Read the model definition and answer for the solid it produces. Units are mm, in the model's axes. Coordinates: 2 decimals unless noted, no trailing zeros. Loops run counter-clockwise (first coordinate to the right, second up) from the corner with the lowest first, then second, coordinate; pieces in that order, holes last.
from build123d import *

# Parameters (mm, degrees)
F0_R     = 5
F1_DEPTH = 10
F2_R     = 2.5
F3_DEPTH = 25
F4_R     = 2.5
F5_DEPTH = 25
F0_R_2   = 2.5
F6_DEPTH = 3


with BuildPart() as f1:
    # F0 (on Front) → F1 (new body)
    with BuildSketch(Plane.XZ):
        with BuildLine():
            Line((-75, 45), (-85, 45))
            Line((-85, 45), (-85, -45))
            Line((-85, -45), (-75, -45))
            Line((-75, -45), (-75, -35))
            Line((-75, -35), (85.1359899874, -35.6216732085))
            ThreePointArc((85.1359899874, -35.6216732085), (120, -0.6219373992), (85.1359899874, 34.3777984101))
            Line((85.1359899874, 34.3777984101), (-75, 35))
            Line((-75, 35), (-75, 45))
        make_face()
        with BuildLine():
            ThreePointArc((87.5, -12.6219373992), (83.232233047, -14.3897043522), (85, -10.1219373992))
            ThreePointArc((85, -10.1219373992), (86.767766953, -10.8541704462), (87.5, -12.6219373992))
        make_face(mode=Mode.SUBTRACT)
        with BuildLine():
            ThreePointArc((85, 3.3780626008), (87.8284271247, 2.2064897255), (89, -0.6219373992))
            ThreePointArc((89, -0.6219373992), (87.8284271247, -3.450364524), (85, -4.6219373992))
            ThreePointArc((85, -4.6219373992), (81, -0.6219373992), (85, 3.3780626008))
        make_face(mode=Mode.SUBTRACT)
        with Locations((-75, 0)):
            Circle(F0_R, mode=Mode.SUBTRACT)
        Circle(F0_R, mode=Mode.SUBTRACT)
        with BuildLine():
            ThreePointArc((87.5, 11.3780626008), (86.767766953, 9.6102956478), (85, 8.8780626008))
            ThreePointArc((85, 8.8780626008), (83.232233047, 13.1458295538), (87.5, 11.3780626008))
        make_face(mode=Mode.SUBTRACT)
    extrude(amount=F1_DEPTH)

    # F2 (on face) → F3 (cut)
    with BuildSketch(Plane.YZ.offset(-75)):
        with Locations((-5, 40)):
            Circle(F2_R)
    extrude(amount=-F3_DEPTH, mode=Mode.SUBTRACT)

    # F4 (on face) → F5 (cut)
    with BuildSketch(Plane.YZ.offset(-75)):
        with Locations((-5, -40)):
            Circle(F4_R)
    extrude(amount=-F5_DEPTH, mode=Mode.SUBTRACT)

    # F0 (on Front) → F6 (join)
    with BuildSketch(Plane.XZ):
        with Locations((-75, 0)):
            Circle(F0_R)
        with Locations((-75, 0)):
            Circle(F0_R_2, mode=Mode.SUBTRACT)
        Circle(F0_R)
        Circle(F0_R_2, mode=Mode.SUBTRACT)
    extrude(amount=F6_DEPTH)


solid = f1.part
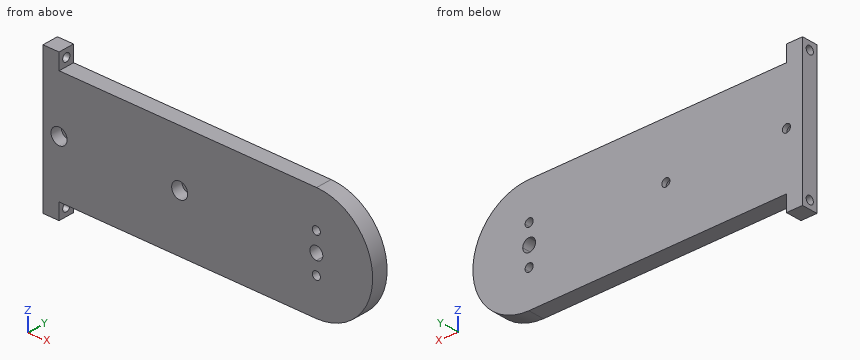
Item 1: Given pin 1 (12 mm diameter, centred on x = 25.5, z = 18.5, fed in from +Y); pin 2 (3 mm diameter, centred on y = -2, z = 25, fed in from +X); pin 3 (6 mm diameter, centred on y = -5, z = 40, fed in from +X), each flat-ended and moving along its own axis, determine where each tip first touches the part or whether it passes through.
Numbers:
pin 1: stops at y = 0
pin 2: stops at x = 110.36
pin 3: stops at x = -75
Item 2: A cutting plane is placed at B-B on z = 40. Determine the outline of the cut face in (x, y).
Numbers:
outline: (-85, -10) - (-75, -10) - (-75, -7.5) - (-85, -7.5) - close; (-85, -2.5) - (-75, -2.5) - (-75, 0) - (-85, 0) - close
Item 3: A cutting plane is placed at C-C on z = -25. Determine the outline of the cut face in (x, y), then the cut area to 3 significant figures.
Numbers:
outline: (-85, -10) - (110.11, -10) - (110.11, 0) - (-85, 0) - close
area: 1,950 mm2
Item 4: A cutting plane is placed at A-A on y = -5. Determine the outline of the cut face in (x, z).
Numbers:
outline: (-85, -45) - (-75, -45) - (-75, -42.5) - (-85, -42.5) - close; (-85, -37.5) - (-75, -37.5) - (-75, -35) - (85.14, -35.62) arc R35 ccw to (85.14, 34.38) - (-75, 35) - (-75, 37.5) - (-85, 37.5) - close; (-85, 42.5) - (-75, 42.5) - (-75, 45) - (-85, 45) - close; hole circle Ø10 at (-75, 0); hole circle Ø10 at (0, 0); hole circle Ø8 at (85, -0.62); hole circle Ø5 at (85, -12.62); hole circle Ø5 at (85, 11.38)
Item 5: A cutting plane is placed at D-D on x = 30.5. Determine the outline of the cut face in (y, z).
Numbers:
outline: (-10, -35.41) - (0, -35.41) - (0, 34.59) - (-10, 34.59) - close
Item 6: Find the intervals of material crossed by line 1 along X through (y, z) = (-4.25, 1.5); line 2 along X through (y, z) = (-8.5, -39); line 3 along Z through (x, y) = (-77.25, -5), in increasing order.
Numbers:
line 1: x = -85 to -79.77, -70.23 to -4.77, 4.77 to 81.61, 88.39 to 119.94
line 2: x = -85 to -75
line 3: z = -45 to -42.5, -37.5 to -4.47, 4.47 to 37.5, 42.5 to 45
